Verification items for this drawing (mm, ordinates from the low corner). A direction names the side the tool comes from. Give positions to 0.01 mm unless a question says otherwise; leave off trailing zeros. Write each loop counter-clockwise with the first axis right and the second up, starting at its lowest first coordinate (ties: lowest second). Pieces come first, ordered by that corner, then holes. Notation, with made-up numbers: (-22, -16) -> (-6, -16) arc R19 cw to (-6, -5) -> close; hole circle Ø10 at (5.5, -6). An arc over 180 degrees is marked (long way). One line per item, written item: value.
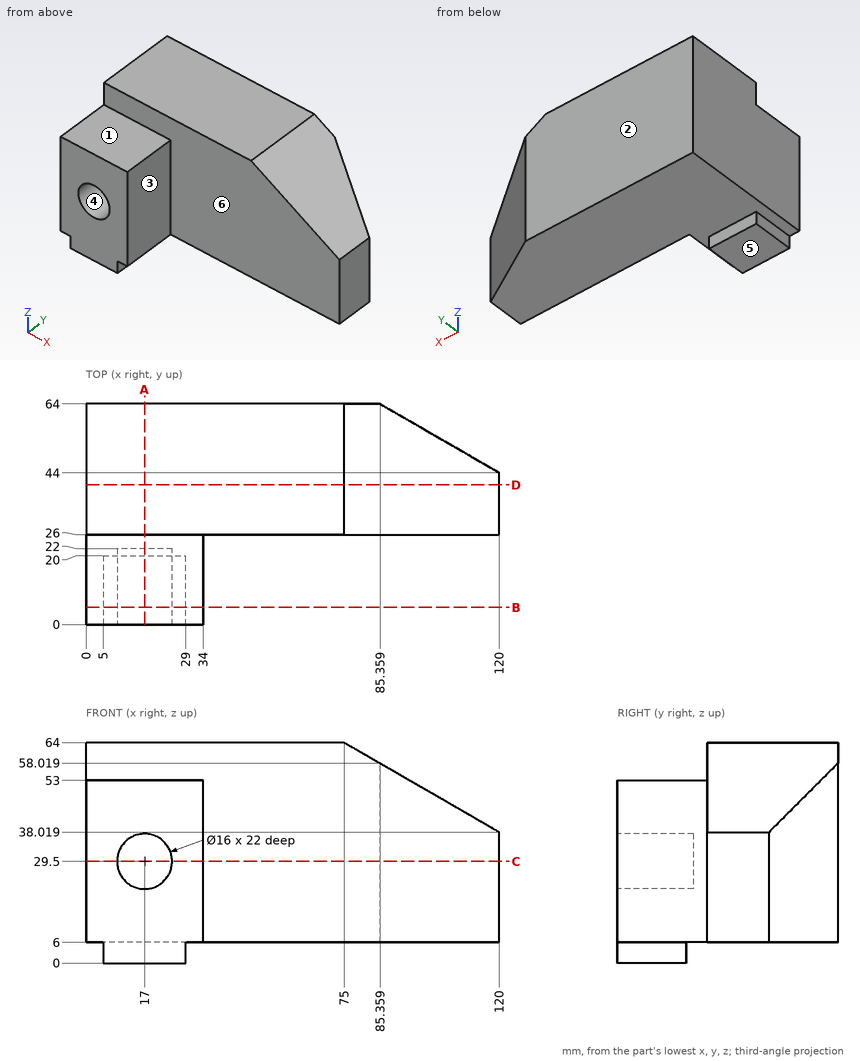
1) Scan lines: probe 1 along X at (y, z) = (7, 29); probe 2 along Z at (x, y) = (17, 5.25); probe 3 along Z at (x, y) = (24.5, 33.5). Record each from-to range of solid material in increasing order.
Verdict:
probe 1: 0 to 9.02, 24.98 to 34
probe 2: 0 to 21.5, 37.5 to 53
probe 3: 6 to 64
2) Sectioned sample at C-C on z = 29.5. Record the cut outline in (x, y), plus the area to 3 significant figures.
Verdict:
outline: (0, 0) -> (9, 0) -> (9, 22) -> (25, 22) -> (25, 0) -> (34, 0) -> (34, 26) -> (120, 26) -> (120, 44) -> (85.36, 64) -> (0, 64) -> close
area: 4,750 mm^2
3) Mould release check, pull along Z, two halves, no side actions. Record for the marked faces 4, 5 and 6: released by +Z, released by -Z, zero draft, split by the parting line, or undercut.
Verdict:
face 4: undercut
face 5: released by -Z
face 6: zero draft
4) Sectioned sample at D-D on y = 40.5. Record the cut outline in (x, z), plus the area to 3 significant figures.
Verdict:
outline: (0, 6) -> (120, 6) -> (120, 38.02) -> (75, 64) -> (0, 64) -> close
area: 6,380 mm^2
5) Tool access check on the marked faces 1, 2 and 3. Record the directions out of +Z, -Z, +X, -X, +Y, -Y that give a thin tool (end or side, any length) a straight path to the whole face; none if there is none.
Verdict:
face 1: +Z, +X, -X, -Y
face 2: +Z, -Z, +X, -X, +Y
face 3: +Z, -Z, +X, -Y
6) Sectioned sample at A-A on x = 17. Record the cut outline in (y, z).
Verdict:
outline: (0, 0) -> (20, 0) -> (20, 6) -> (64, 6) -> (64, 64) -> (26, 64) -> (26, 53) -> (0, 53) -> (0, 37.5) -> (22, 37.5) -> (22, 21.5) -> (0, 21.5) -> close
7) Depth check by flat-ended pin: pin 1 Ø1.8 at (x, z) = (22, 4) entering from +Y; pin 2 Ø8 at (y, z) = (6.5, 22) entering from +X; pin 3 Ø1.8 at (y, z) = (12.5, 3.5) entering from -X. Enter the tip coordinate at first touch or a pass-through.
Verdict:
pin 1: y = 20
pin 2: x = 34
pin 3: x = 5
8) Sectioned sample at B-B on y = 5. Record the cut outline in (x, z).
Verdict:
outline: (0, 6) -> (5, 6) -> (5, 0) -> (29, 0) -> (29, 6) -> (34, 6) -> (34, 53) -> (0, 53) -> close; hole circle Ø16 at (17, 29.5)
